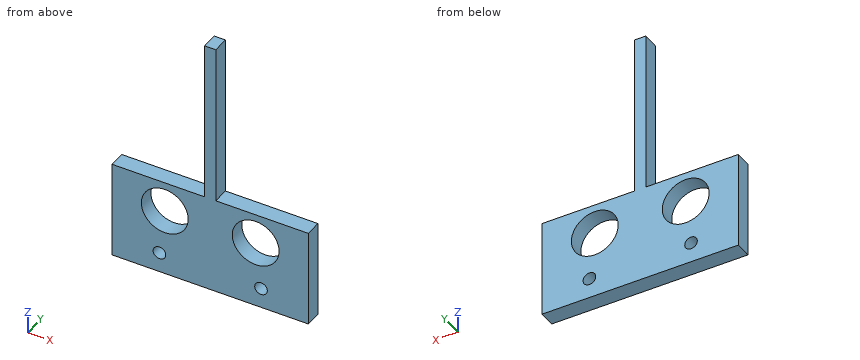
```python
from build123d import *

# Parameters (mm, degrees)
F0_W     = 4.335432
F0_H     = 63.5
F0_R     = 2.4511
F0_R_2   = 9.0932
F1_DEPTH = 6.35


with BuildPart() as f1:
    # F0 (on Front) → F1 (new body)
    with BuildSketch(Plane.XZ):
        with Locations((0, 50.8)):
            Rectangle(F0_W, F0_H)
        Polygon((-38.1, -19.05), (38.1, -19.05), (38.1, 19.05), (2.167716, 19.05), (-2.167716, 19.05), (-38.1, 19.05), align=None)
        with Locations((-19.731838, -11.16004)):
            Circle(F0_R, mode=Mode.SUBTRACT)
        with Locations((-17.65278, 7.1953)):
            Circle(F0_R_2, mode=Mode.SUBTRACT)
        with Locations((19.731838, -11.16004)):
            Circle(F0_R, mode=Mode.SUBTRACT)
        with Locations((17.65278, 7.1953)):
            Circle(F0_R_2, mode=Mode.SUBTRACT)
    extrude(amount=F1_DEPTH)


solid = f1.part
```
Here's how the part is built. I have some questions about the finished solid (model axes, mm). Coordinates: 2 decimals unless noted, no trailing zeros. Order: outer loops, then holes, each group sorted by start corner. A loop starts at its lowest first (then second) coordinate and runs counter-clockwise, first axis right, second up. Notation, with made-up numbers: (-7.75, 64.25) - (30.25, 64.25) arc R12 cw to (30.25, 84.25) - close; hole circle Ø2 at (19, 84.25). An arc over 180 degrees is marked (long way). One line per question, with ' | ' between items. Start each with the question number.
1. If we section it at B-B (y = -3.5): Write out the boundary of the cut face in (x, z).
2. I'm going to push flat-ended pins straight in: pin 1 Ø1.9 at (x, y) = (-14, -2.5) entering from +Z; pin 2 Ø1.9 at (y, z) = (-2.5, 41.5) entering from -X. Where does each tip first touch, or does it pass through?
3. If we section it at A-A (z = 4): Write out the boundary of the cut face in (x, y).
4. Please list where these lines run through material, in increasing order: line 1 along Z through (x, y) = (-17, -0.25); line 2 along Z through (x, y) = (-18, -1); line 3 along Z through (x, y) = (-20, -3.75). Write a range as [from, to].
5. If we section it at C-C (x = 25): Write out the boundary of the cut face in (y, z), and give its area (3 significant figures).
6. If we section it at D-D (x = 3.5): Write out the boundary of the cut face in (y, z).
Model answer:
1) outline: (-38.1, -19.05) - (38.1, -19.05) - (38.1, 19.05) - (2.17, 19.05) - (2.17, 82.55) - (-2.17, 82.55) - (-2.17, 19.05) - (-38.1, 19.05) - close; hole circle Ø18.19 at (-17.65, 7.2); hole circle Ø4.9 at (-19.73, -11.16); hole circle Ø18.19 at (17.65, 7.2); hole circle Ø4.9 at (19.73, -11.16)
2) pin 1: stops at z = 19.05 | pin 2: stops at x = -2.17
3) outline: (-38.1, -6.35) - (-26.17, -6.35) - (-26.17, 0) - (-38.1, 0) - close; (-9.14, -6.35) - (9.14, -6.35) - (9.14, 0) - (-9.14, 0) - close; (26.17, -6.35) - (38.1, -6.35) - (38.1, 0) - (26.17, 0) - close
4) line 1: z = [-19.05, -1.87], [16.27, 19.05] | line 2: z = [-19.05, -12.89], [-9.43, -1.89], [16.28, 19.05] | line 3: z = [-19.05, -13.6], [-8.72, -1.59], [15.98, 19.05]
5) outline: (-6.35, -19.05) - (0, -19.05) - (0, 1.84) - (-6.35, 1.84) - close; (-6.35, 12.55) - (0, 12.55) - (0, 19.05) - (-6.35, 19.05) - close | area: 174 mm²
6) outline: (-6.35, -19.05) - (0, -19.05) - (0, 19.05) - (-6.35, 19.05) - close
